Input: dimensioned drawing with shaded views. Units: mm. Origin: part minimum x, y, z. A direction names the side the tool comes from. Coordinates: 2 decimals unless noted, no trailing zeros. Loops run counter-clockwise (first coordinate to the right, second up) from the corner with the lowest first, then second, coordinate; pieces in that order, holes last.
Item 1: Section query C-C, the plane z = 14.5. Return the cut outline in (x, y).
Item 2: Line query: probe 1 along Z at (x, y) = (9.5, 3); probe 2 along Y at (x, z) = (7, 10.5); probe 3 along X at (y, z) = (8.75, 12.75). Output: solid intervals per line, ascending.
Item 3: Section query D-D, the plane z = 3.25. Return the cut outline in (x, y).
Item 4: Pin query (flat end, axial travel): pin 1 Ø4 at (x, z) = (8, 6) entering from -Y; pin 2 Ø1 at (x, z) = (5.5, 9) entering from +Y; pin 3 Ø6 at (y, z) = (3.5, 2.5) entering from +X. Return the tip coordinate at first contact, or that it passes through.
Item 5: Section query A-A, the plane x = 7. Return the cut outline in (y, z), then the cut area to 3 significant figures.
Item 6: Reachability of the marked faces 5 and 6 from +Z, -Z, +X, -X, +Y, -Y: full face, straight path, thin tool, end or side. Return the list, or none.
Item 7: Pull-direction query (Z, two-part tool) for the marked faces 1, 2, 3 and 4; classes: +Z half, -Z half, draft (parallel to the pull), parting line (faces both ways), or undercut.
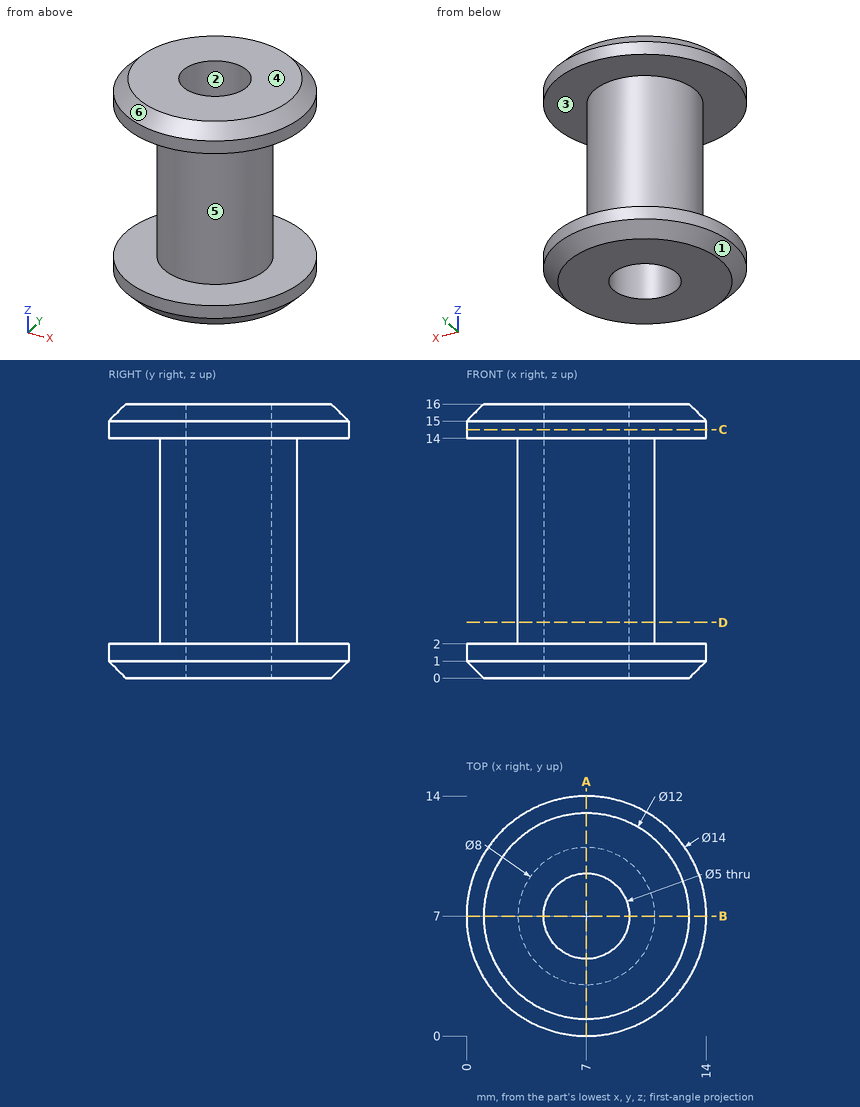
Verdict:
1. outline: circle Ø14 at (7, 7); hole circle Ø5 at (7, 7)
2. probe 1: z = 0 to 2, 14 to 16
2. probe 2: y = 3 to 4.5, 9.5 to 11
2. probe 3: x = 3.4 to 5.21, 8.79 to 10.6
3. outline: circle Ø8 at (7, 7); hole circle Ø5 at (7, 7)
4. pin 1: stops at y = 3
4. pin 2: stops at y = 10.87
4. pin 3: stops at x = 13.98
5. outline: (0, 1) - (1, 0) - (4.5, 0) - (4.5, 16) - (1, 16) - (0, 15) - (0, 14) - (3, 14) - (3, 2) - (0, 2) - close; (9.5, 0) - (13, 0) - (14, 1) - (14, 2) - (11, 2) - (11, 14) - (14, 14) - (14, 15) - (13, 16) - (9.5, 16) - close
5. area: 70.0 mm2
6. face 5: none
6. face 6: +Z
7. face 1: -Z half
7. face 2: draft
7. face 3: undercut
7. face 4: +Z half
